```python
from build123d import *

# Parameters (mm, degrees)
EXTRUDE006_START = -0.7
SKETCH006_W      = 4
SKETCH006_H      = 1
EXTRUDE006_DEPTH = 0.5
FILLET001_R      = 0.4
SKETCH005_W      = 16
SKETCH005_H      = 1
EXTRUDE005_DEPTH = 1.2
EXTRUDE004_DEPTH = 2
SKETCH002_R      = 2.2
EXTRUDE002_DEPTH = 2.8
SKETCH007_W      = 6
SKETCH007_H      = 1.5
EXTRUDE007_DEPTH = 0.3
EXTRUDE001_START = -0.2
SKETCH001_W      = 6
SKETCH001_H      = 3
EXTRUDE001_DEPTH = 1
FILLET_R         = 0.9
SKETCH_W         = 26
SKETCH_H         = 15.5
EXTRUDE_DEPTH    = 1.2


with BuildPart() as fillet001:
    # Sketch006 → Extrude006 (new body)
    with BuildSketch(Plane.XY.offset(EXTRUDE006_START)):
        with Locations((12.75, 0)):
            Rectangle(SKETCH006_W, SKETCH006_H)
    extrude(amount=-EXTRUDE006_DEPTH)

    # Fillet001
    fillet001_edges = [fillet001.edges().sort_by_distance(p)[0] for p in [
        (12.75, -0.5, -1.2),
    ]]
    fillet(fillet001_edges, radius=FILLET001_R)


with BuildPart() as extrude005:
    # Sketch005 → Extrude005 (new body)
    with BuildSketch(Plane.XY):
        with Locations((13, 0.5)):
            Rectangle(SKETCH005_W, SKETCH005_H)
    extrude(amount=-EXTRUDE005_DEPTH)


with BuildPart() as extrude004:
    # Sketch004 → Extrude004 (new body)
    with BuildSketch(Plane.XY):
        with BuildLine():
            ThreePointArc((6, 2), (5.5, 1.5), (6, 1))
            Line((6, 1), (20, 1))
            ThreePointArc((20, 1), (20.5, 1.5), (20, 2))
            Line((6, 2), (20, 2))
        make_face()
    extrude(amount=EXTRUDE004_DEPTH)


with BuildPart() as extrude002:
    # Sketch002 → Extrude002 (new body)
    with BuildSketch(Plane.XY):
        with Locations((2.5, 2.5)):
            Circle(SKETCH002_R)
        with Locations((23.5, 2.5)):
            Circle(SKETCH002_R)
    extrude(amount=-EXTRUDE002_DEPTH)


with BuildPart() as extrude007:
    # Sketch007 (on Fillet) → Extrude007 (new body)
    with BuildSketch(Plane.XY):
        with Locations((6.5, 14.75)):
            Rectangle(SKETCH007_W, SKETCH007_H)
        with Locations((19.5, 14.75)):
            Rectangle(SKETCH007_W, SKETCH007_H)
    extrude(amount=-EXTRUDE007_DEPTH)


with BuildPart() as fusion005:
    # Sketch001 (on Sketch) → Extrude001 (new body)
    with BuildSketch(Plane.XY.offset(EXTRUDE001_START)):
        with Locations((6.5, 15.5)):
            Rectangle(SKETCH001_W, SKETCH001_H)
        with Locations((19.5, 15.5)):
            Rectangle(SKETCH001_W, SKETCH001_H)
    extrude(amount=-EXTRUDE001_DEPTH)

    # Fillet
    fillet_edges = [fusion005.edges().sort_by_distance(p)[0] for p in [
        (19.5, 17, -1.2),
        (19.5, 14, -1.2),
        (6.5, 17, -1.2),
        (6.5, 14, -1.2),
    ]]
    fillet(fillet_edges, radius=FILLET_R)

    # Fusion005: union Extrude007
    add(extrude007.part)


with BuildPart() as fusion004:
    # Sketch → Extrude (new body)
    with BuildSketch(Plane.XY):
        with Locations((13, 7.75)):
            Rectangle(SKETCH_W, SKETCH_H)
    extrude(amount=EXTRUDE_DEPTH)

    # Fusion: union Fusion005
    add(fusion005.part)

    # Fusion001: union Extrude002
    add(extrude002.part)

    # Cut001: cut Extrude004
    add(extrude004.part, mode=Mode.SUBTRACT)

    # Fusion003: union Extrude005
    add(extrude005.part)

    # Fusion004: union Fillet001
    add(fillet001.part)


solid = fusion004.part
```
The listing builds one solid part. Answer for the finished solid, in the listing's coordinates (mm). A direction names the side the tool comes from. Give positions to 0.01 mm unless a question says otherwise; leave off trailing zeros. Order: outer loops, then holes, each group sorted by start corner. A loop starts at its lowest first (then second) coordinate and runs counter-clockwise, first axis right, second up.
Item 1: The part is cut by section B-B, the plane y = 1.5. Give the vertices of the cut face in (x, z).
From the geometry:
outline: (0, 0) - (0.54, 0) - (0.54, -2.8) - (4.46, -2.8) - (4.46, 0) - (5.5, 0) - (5.5, 1.2) - (0, 1.2) - close; (20.5, 0) - (21.54, 0) - (21.54, -2.8) - (25.46, -2.8) - (25.46, 0) - (26, 0) - (26, 1.2) - (20.5, 1.2) - close
Item 2: The part is cut by section C-C, the plane z = -2. Give the vertices of the cut face in (x, y), and give its area (3 significant figures).
From the geometry:
outline: circle Ø4.4 at (2.5, 2.5); circle Ø4.4 at (23.5, 2.5)
area: 30.4 mm2
Item 3: Given pin 1 Ø0.6 at (x, y) = (10.5, 0.5) entering from -Z; pin 2 Ø0.5 at (y, z) = (0.5, -0.5) entering from -X; pin 3 Ø1 at (y, z) = (15.5, -1) entering from -X; pin 4 Ø1.5 at (y, z) = (12.5, 0.5) entering from -X, each flat-ended and moving along its own axis, determine where each tip first touches the part or whether it passes through.
From the geometry:
pin 1: stops at z = -1.2
pin 2: stops at x = 1.17
pin 3: stops at x = 3.5
pin 4: stops at x = 0
Item 4: Find the intervals of material crossed by probe 1 along Y at (x, z) = (8.25, 0.8); probe 2 along Z at (x, y) = (4.5, 5.5); probe 3 along Y at (x, z) = (13, -0.85), in increasing order.
From the geometry:
probe 1: y = 0 to 1, 2 to 15.5
probe 2: z = 0 to 1.2
probe 3: y = -0.5 to 1
Item 5: The part is cut by section A-A, the plane x = 18.5. Give the vertices of the cut face in (y, z), and give its area (3 significant figures).
From the geometry:
outline: (0, -1.2) - (1, -1.2) - (1, 1.2) - (0, 1.2) - close; (2, 0) - (14, 0) - (14, -0.3) arc R0.9 ccw to (14.9, -1.2) - (16.1, -1.2) arc R0.9 ccw to (17, -0.3) - (17, -0.2) - (15.5, -0.2) - (15.5, 1.2) - (2, 1.2) - close
area: 21.6 mm2
Item 6: For a pull along X with two mould halves and no side action, classify faces 6 (the face through (13, 8, 0)), 7 (the face through (3.5, 15, -1)), 8 (the face through (19.54, 16.74, -0.93)) as pulls with the +X half, pulls with the -X half, needs draft (parallel to the pull), parting line crosses it, or undercut.
From the geometry:
face 6: undercut
face 7: pulls with the -X half
face 8: needs draft
Item 7: The part is cut by section D-D, the plane x = 23.5. Give the vertices of the cut face in (y, z).
From the geometry:
outline: (0, 0) - (0.3, 0) - (0.3, -2.8) - (4.7, -2.8) - (4.7, 0) - (15.5, 0) - (15.5, 1.2) - (0, 1.2) - close
Item 8: Which of the six approach directions +Z, -Z, +X, -X, +Y, -Y give full straight-line access (tool end or side, diameter ignored) to faces 1 (the face through (16.5, 15, -1)), 2 (the face through (5.5, 1.5, 0.6)), 3 (the face through (6.5, 15.5, -1.2)), 4 (the face through (12.8, 15.5, 0.5)), 5 (the face through (2.21, 4.68, -1.38))?
From the geometry:
face 1: -Z, +Y
face 2: +Z, -Z
face 3: -Z, +X, -X, +Y
face 4: +Z, +X, -X, +Y
face 5: -Z
